Part model, mm, in its own coordinate system. A direction names the side the tool comes from. Round coordinates to 2 decimals unless told otherwise and drop trailing zeros. Write each loop counter-clockwise with the first axis right and the second up, starting at its lowest first coordinate (ties: lowest second). Pieces come first, ordered by that corner, then holes. Notation, with made-up numbers: (76.5, 1) -> (81.5, 1) arc R24 ccw to (81.5, 34) -> close; hole circle Ø11 at (2.5, -31). An arc over 180 degrees is marked (long way). Use CSV: the item, a comma, the result in double quotes. Start each with the question number.
(1) Saw through at B-B (y = 133). Give the cut face in (x, z), plus the area to 3 significant figures.
(2) Saw through at D-D (x = 48.5). Give the cut face in (y, z), plus the area to 3 significant figures.
(3) Probe line 1 (X direction, y = 133, z = 1.5); line 2 (Y direction, x = 50, z = 20); line 3 (Y direction, x = 8, z = 4.5). List the from-to ranges inside material, lowest first. Write a range as [from, to].
(4) Saw through at A-A (x = 8). Give the cut face in (y, z), plus the area to 3 significant figures.
(5) Drop flat-ended pins along their axis: pin 1 (9 mm diameter, centred on y = 118, z = 13, fed in from -X); pin 2 (10 mm diameter, centred on y = 126.5, z = 9, fed in from -X); pin 3 (5 mm diameter, centred on y = 138.3, z = 20, fed in from +X); pin 4 (6.5 mm diameter, centred on x = 21, z = 5, fed in from -Y). Give the stop position or say it passes through.
(6) Which spindle directions (+Z, -Z, +X, -X, +Y, -Y) get a long thin tool onto all of the face, cutting with end or side? Do faces 5 (the flat face through (21, 118, 4)), 6 (the flat face through (47, 123, 30)), 7 (the flat face through (21, 133, 8)). Say none if no direction does.
(7) Two-plate mould, pull along Z, no slides. Class faces 1 (the cylindrical face through (47.07, 103.615, 20.596)), 2 (the cylindrical face through (47.07, 135.615, 20.596)), 3 (the cylindrical face through (33.67, 135.48, 4.06)), 4 (the flat face through (31, 129, 0)): released by +Z, released by -Z, zero draft, split by the parting line, or undercut.
(8) Saw through at C-C (y = 106.3). Give the cut face in (x, z), plus the area to 3 significant figures.
```python
from build123d import *

# Parameters (mm, degrees)
SKETCH1_W             = 42
SKETCH1_H             = 30
BOSS_EXTRUDE1_DEPTH   = 8
BOSS_EXTRUDE1_2_DEPTH = 8
BOSS_EXTRUDE2_DEPTH   = 30
SKETCH2_R             = 2.5
CUT_EXTRUDE1_DEPTH    = 8
SKETCH3_R             = 2.75
CUT_EXTRUDE2_DEPTH    = 10
SKETCH6_W             = 30
SKETCH6_H             = 97
CUT_EXTRUDE6_DEPTH    = 52


with BuildPart() as part:
    # Sketch1 → Boss-Extrude1 (new body)
    with BuildSketch(Plane.XY):
        with Locations((21, 133)):
            Rectangle(SKETCH1_W, SKETCH1_H)
    extrude(amount=BOSS_EXTRUDE1_DEPTH)



with BuildPart() as body_2:
    # Sketch1 → Boss-Extrude1 2 (new body)
    with BuildSketch(Plane.XY):
        with Locations((21, 15)):
            Rectangle(SKETCH1_W, SKETCH1_H)
    extrude(amount=BOSS_EXTRUDE1_2_DEPTH)


with BuildPart() as part_1:
    add(part.part)

    add(body_2.part)  # Boss-Extrude2 merges body 2
    # Sketch1<3> → Boss-Extrude2 (add)
    with BuildSketch(Plane.XY):
        Polygon((42, 30), (42, 0), (52, 0), (52, 148), (42, 148), (42, 118), align=None)
    extrude(amount=BOSS_EXTRUDE2_DEPTH)

    # Sketch2 → Cut-Extrude1 (cut)
    with BuildSketch(Plane.XY.offset(8)):
        with Locations((8, 133)):
            Circle(SKETCH2_R)
        with Locations((34, 133)):
            Circle(SKETCH2_R)
        with Locations((34, 15)):
            Circle(SKETCH2_R)
        with Locations((8, 15)):
            Circle(SKETCH2_R)
    extrude(amount=-CUT_EXTRUDE1_DEPTH, mode=Mode.SUBTRACT)

    # Sketch3 → Cut-Extrude2 (cut)
    with BuildSketch(Plane(origin=(52, 0, 0), x_dir=(0, 0, -1), z_dir=(1, 0, 0))):
        with Locations((-20, 138.3)):
            Circle(SKETCH3_R)
        with Locations((-20, 106.3)):
            Circle(SKETCH3_R)
        with Locations((-20, 41.2)):
            Circle(SKETCH3_R)
        with Locations((-20, 9.2)):
            Circle(SKETCH3_R)
    extrude(amount=-CUT_EXTRUDE2_DEPTH, mode=Mode.SUBTRACT)

    # Sketch6 → Cut-Extrude6 (cut)
    with BuildSketch(Plane.ZY):
        with Locations((15, 48.5)):
            Rectangle(SKETCH6_W, SKETCH6_H)
    extrude(amount=-CUT_EXTRUDE6_DEPTH, mode=Mode.SUBTRACT)


solid = part_1.part
```
Answers:
1,outline,"(0, 0) -> (5.5, 0) -> (5.5, 8) -> (0, 8) -> close; (10.5, 0) -> (31.5, 0) -> (31.5, 8) -> (10.5, 8) -> close; (36.5, 0) -> (52, 0) -> (52, 30) -> (42, 30) -> (42, 8) -> (36.5, 8) -> close"
1,area,"556 mm²"
2,outline,"(97, 0) -> (148, 0) -> (148, 30) -> (97, 30) -> close; hole circle Ø5.5 at (106.3, 20); hole circle Ø5.5 at (138.3, 20)"
2,area,"1,480 mm²"
3,line 1,"x = [0, 5.5], [10.5, 31.5], [36.5, 52]"
3,line 2,"y = [97, 103.55], [109.05, 135.55], [141.05, 148]"
3,line 3,"y = [118, 130.5], [135.5, 148]"
4,outline,"(118, 0) -> (130.5, 0) -> (130.5, 8) -> (118, 8) -> close; (135.5, 0) -> (148, 0) -> (148, 8) -> (135.5, 8) -> close"
4,area,"200 mm²"
5,pin 1,"stops at x = 42"
5,pin 2,"stops at x = 0"
5,pin 3,"passes through"
5,pin 4,"stops at y = 118"
6,face 5,"+Z, -Z, -X, -Y"
6,face 6,"+Z, +X, -X, +Y, -Y"
6,face 7,"+Z, -X, +Y, -Y"
7,face 1,"undercut"
7,face 2,"undercut"
7,face 3,"zero draft"
7,face 4,"released by -Z"
8,outline,"(42, 0) -> (52, 0) -> (52, 17.25) -> (42, 17.25) -> close; (42, 22.75) -> (52, 22.75) -> (52, 30) -> (42, 30) -> close"
8,area,"245 mm²"
